Input: part model. Units: mm. Frame: model coordinates. A direction names the side the tool comes from. Coordinates: 2 decimals unless noted, no trailing zeros. Write each loop counter-clockwise with the first axis right and the second up, starting at its lowest first coordinate (ties: lowest second). Pieces come first, ordered by that corner, then holes. Notation, with made-up numbers: (-18, 43.5) - (30, 43.5) arc R11 ccw to (30, 52.5) - close; hole circle Ø5 at (18, 6). An arc over 180 degrees is marked (long way). Put each result on its own line as item: value. Start each with the question number.
1. Cut plane B-B, the plane x = -31. Return loops of the section in (y, z).
2. Line query: line 1 (X direction, y = 11.5, z = 4); line 2 (X direction, y = 9.5, z = 2); line 3 (Z direction, x = -69, y = 2). Output: solid intervals per line, ascending.
3. Pull-direction query (Y, two-part tool) for faces 1 (the flat face through (68, 0, 3.5)), 2 (the flat face through (-17.5, 3, -10)), 3 (the cylindrical face through (17.08, -7.493, -0.33)); classes: released by +Y, released by -Y, zero draft, split by the parting line, or undercut.
4. Access query for faces 4 (the flat face through (47.5, 2, 6)), 5 (the flat face through (-85.5, 0, 0)), 6 (the cylindrical face through (-34.23, -2.17, 9.76)), 7 (the flat face through (-61, 0, 5)). Directions: +Z, -Z, +X, -X, +Y, -Y. A direction counts if a zero-diameter tool reaches every point of the face in a straight line with its end or side. Return the directions, or none.
5. Cut plane D-D, the plane x = -57.5. Return loops of the section in (y, z).
6. Pin query (flat end, axial travel): pin 1 (2 mm diameter, centred on x = -45.5, y = -4, fed in from -Z); pin 2 (1.5 mm diameter, centred on x = -37, z = 11, fed in from +Y); pin 3 (5.5 mm diameter, centred on x = -60, y = 1, fed in from +Z); pin 4 (10 mm diameter, centred on x = -53.5, z = -7.5, fed in from -Y). Return the tip coordinate at first contact, or that it passes through.
7. Cut plane C-C, the plane x = -9.5. Return loops of the section in (y, z).
8. Cut plane A-A, the plane z = 0. Return loops of the section in (x, y), and give its area (3 significant figures).
Autodesk Inventor part; units mm, degrees
ref_plane "Work Plane2" through (-68, 0, 8) normal (0, 0, 1) x (1, 0, 0)
ref_plane "YZ Plane" through (0, 0, 0) normal (1, 0, 0) x (0, 1, 0)
ref_plane "XZ Plane" through (0, 0, 0) normal (0, 1, 0) x (-1, 0, 0)
sketch "Sketch1" plane through (0, 0, 0) normal (0, 0, 1) x (1, 0, 0)
  line L0 (-85.5, 0) -> (85.5, 0)
  line L1 (85.5, 0) -> (85.5, 6)
  line L2 (85.5, 6) -> (47.5, 6)
  line L3 (47.5, 6) -> (47.5, 7.5)
  line L4 (47.5, 7.5) -> (-12.5, 7.5)
  line L5 (-12.5, 7.5) -> (-12.5, 15)
  line L6 (-12.5, 15) -> (-17.5, 15)
  line L7 (-17.5, 15) -> (-17.5, 10)
  line L8 (-17.5, 10) -> (-50.5, 10)
  line L9 (-85.5, 0) -> (-85.5, 8)
  line L10 (-85.5, 8) -> (-50.5, 8)
  line L11 (-50.5, 10) -> (-50.5, 8)
  point P0 (0, 0)
  point P1 (0, 0)
  dimension "d8" = 12
  dimension "d9" = 15
  dimension "d10" = 30
  dimension "d11" = 20
  dimension "d12" = 98
  dimension "d13" = 5
  dimension "d14" = 60
  dimension "d15" = 33
  dimension "d16" = 16
  dimension "d43" = 68
revolve "Revolution1" add sketch "Sketch1" angle 360 about axis through (-85.5, 0, 0) along (1, 0, 0)
thread "Thread1"
chamfer "Chamfer1" distance 1 angle 45 2 edges at (85.5, -6, 0) (-85.5, -8, 0)
sketch "Sketch4" plane through (85.5, 0, 0) normal (1, 0, 0) x (0, 0, -1)
  circle A0 centre (0, 0) radius 6
  line L0 (-5.6569, -2) -> (-3.5, -2)
  line L1 (-3.5, -2) -> (-3.5, 2)
  line L2 (-3.5, 2) -> (-5.6569, 2)
  point P0 (0, 0)
  dimension "d35" = 9.5
  dimension "d36" = 4
extrude "Extrusion3" cut sketch "Sketch4" against normal blind 35 contours L2 L1 L0 A0 picked at (-4.3205, -0.2261)
full round fillet "Full Round Fillet1" first side at (73.5, -2, 4.219) centre faces at (50.5, 0.2261, 4.3205) second side at (73.5, 2, 4.219)
thread "Thread2"
ref_plane "Work Plane2" through (-68, 0, 8) normal (0, 0, 1) x (1, 0, 0)
sketch "Sketch3" plane through (-68, 0, 8) normal (0, 0, 1) x (1, 0, 0)
  line L0 (14, -2.5) -> (1, -2.5)
  arc A0 (1, 2.5) -> (1, -2.5) centre (1, 0) ccw
  line L1 (1, 2.5) -> (14, 2.5)
  arc A1 (14, -2.5) -> (14, 2.5) centre (14, 0) ccw
  line L2 (-51.7, 0) -> (187.7, 0)
  line L3 (-17.5, -7) -> (-17.5, 7)
  point P0 (68, 0)
  point P1 (16.5, 0)
  point P2 (-1.5, 0)
  dimension "d40" = 18
  dimension "d41" = 5
  dimension "d42" = 16
extrude "Extrusion2" cut sketch "Sketch3" against normal blind 3
properties material "Steel, Alloy"
Report:
1. outline: circle Ø20 at (0, 0)
2. line 1: x = -17.5 to -12.5
2. line 2: x = -50.5 to -12.5
2. line 3: z = -7.75 to 7.75
3. face 1: undercut
3. face 2: zero draft
3. face 3: split by the parting line
4. face 4: +X
4. face 5: +Z, -Z, -X, +Y, -Y
4. face 6: -X
4. face 7: +Z
5. outline: (-2.5, 5) - (-2.5, 7.6) arc R8 ccw (long way) to (2.5, 7.6) - (2.5, 5) - close
6. pin 1: stops at z = -9.54
6. pin 2: passes through
6. pin 3: stops at z = 7.6
6. pin 4: stops at y = -9.37
7. outline: circle Ø15 at (0, 0)
8. outline: (-85.5, -7) - (-84.5, -8) - (-50.5, -8) - (-50.5, -10) - (-17.5, -10) - (-17.5, -15) - (-12.5, -15) - (-12.5, -7.5) - (47.5, -7.5) - (47.5, -6) - (84.5, -6) - (85.5, -5) - (85.5, 5) - (84.5, 6) - (47.5, 6) - (47.5, 7.5) - (-12.5, 7.5) - (-12.5, 15) - (-17.5, 15) - (-17.5, 10) - (-50.5, 10) - (-50.5, 8) - (-84.5, 8) - (-85.5, 7) - close
8. area: 2,720 mm^2
